Input: dimensioned drawing with shaded views. Units: mm. Origin: part minimum x, y, z. A direction names the side the tool comes from. Round coordinates to 2 decimals unless told otherwise and drop trailing zeros. Order: outer loops, then holes, each group sorted by start corner. A loop starts at its lowest first (then second) coordinate and runs counter-clockwise, first axis right, second up. Notation, with made-up numbers: (25.25, -7) - (74.25, -7) arc R26 cw to (74.25, 8) - close; hole circle Ø5 at (69.25, 58.5). An arc over 180 degrees is marked (long way). Return JSON: item names as keys, results as strings. Group by question number.
1) Section C-C, the plane x = 94. Return loops of the section in (y, z).
2) Section A-A, the plane z = 17. Return loops of the section in (x, y), plus the area to 3 significant figures.
3) Mould query, pull axis X, two halves, no side actions, for the marked faces 1, 2 and 3. Classes: pulls with the +X half, pulls with the -X half, needs draft (parallel to the pull), parting line crosses it, or undercut.
4) Access query for the marked faces 4, 5 and 6. Directions: +Z, -Z, +X, -X, +Y, -Y. A direction counts if a zero-diameter tool reaches every point of the face in a straight line with its end or side. Return the directions, or none.
5) Contact query for flat-ended pins moving along their axis: P1, Ø11.5, axis at x = 4, y = 24.5, coming from the -Z side; P2, Ø6.5, axis at x = 130, y = 22, coming from the +Z side; P3, Ø2, axis at x = 72, z = 38, coming from the +Y side. Output: stop coordinate, or through.
6) Ray query, line 1 (X direction, y = 42.5, z = 2); line 2 (Y direction, x = 57.5, z = 18.5). Return the intervals inside material, ascending. Write a range as from..to.
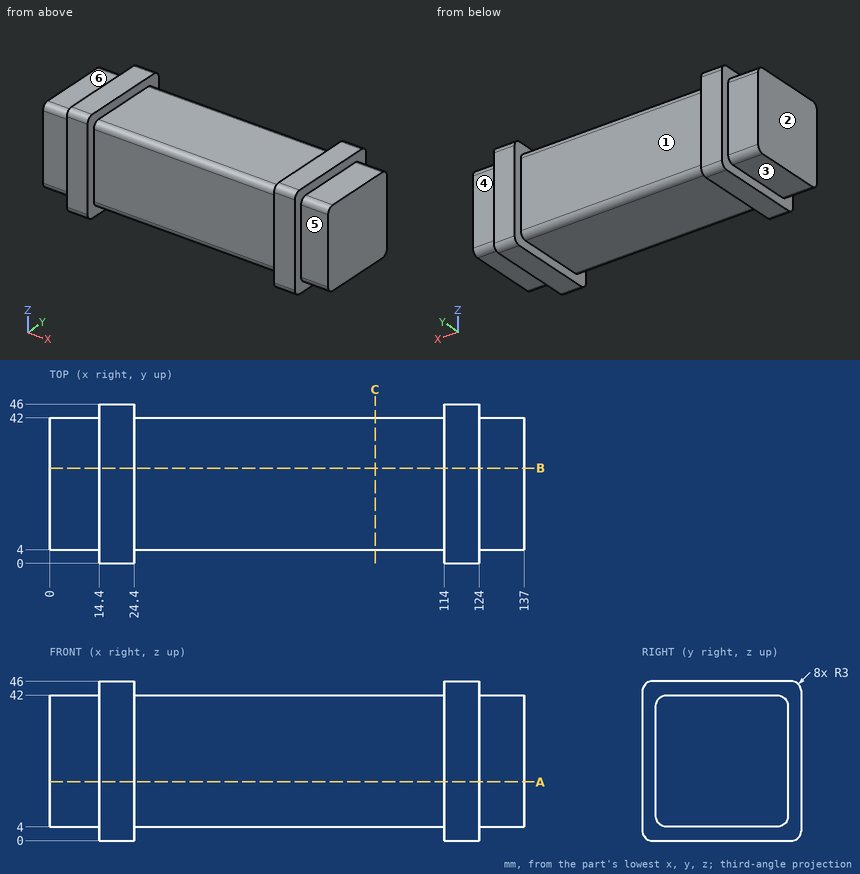
Geometry check:
{
 "1": {"outline": "(4, 7) arc R3 ccw to (7, 4) - (39, 4) arc R3 ccw to (42, 7) - (42, 39) arc R3 ccw to (39, 42) - (7, 42) arc R3 ccw to (4, 39) - close"},
 "2": {"outline": "(0, 4) - (14.4, 4) - (14.4, 0) - (24.4, 0) - (24.4, 4) - (114, 4) - (114, 0) - (124, 0) - (124, 4) - (137, 4) - (137, 42) - (124, 42) - (124, 46) - (114, 46) - (114, 42) - (24.4, 42) - (24.4, 46) - (14.4, 46) - (14.4, 42) - (0, 42) - close", "area": "5,370 mm2"},
 "3": {"face 1": "undercut", "face 2": "pulls with the -X half", "face 3": "needs draft"},
 "4": {"face 4": "+Z, -Z, +X, +Y", "face 5": "+Z, -Z, +X, -Y", "face 6": "+Z, -X, +Y, -Y"},
 "5": {"P1": "z = 4", "P2": "z = 42", "P3": "y = 42"},
 "6": {"line 1": "14.4..24.4, 114..124", "line 2": "4..42"}
}
